Source: CAD feature listing. Evaluate the final solid. Frame: model axes, mm. A direction names the side the tool comes from. Round coordinates to 2 decimals unless told otherwise and drop trailing zeros. Loops run counter-clockwise (first coordinate to the right, second up) from the corner with the lowest first, then second, coordinate; pieces in that order, holes last. Notation, with made-up numbers: (47, -28.75) -> (92, -28.75) arc R36 ccw to (92, 7.25) -> close; hole circle Ø2 at (6, 52). An arc over 180 degrees is marked (long way). Write item = value, one per line.
from build123d import *

# Parameters (mm, degrees)
SKETCH1_R          = 48.5
SKETCH1_R_2        = 27.5
BASE_EXTRUDE_DEPTH = 8


with BuildPart() as part:
    # Sketch1 → Base-Extrude (new body)
    with BuildSketch(Plane.XY):
        with BuildLine():
            Line((456.811048982, 62.151395165), (445.137482247, 71.222327839))
            ThreePointArc((445.137482247, 71.222327839), (408.071209791, 86.463783058), (368.448599855, 80.442214094))
            ThreePointArc((368.448599855, 80.442214094), (344.491847052, 80.189853314), (327.989727135, 97.558495432))
            Line((327.989727135, 97.558495432), (324.860948055, 106.154745303))
            ThreePointArc((324.860948055, 106.154745303), (311.314649231, 123.808625639), (290.092321086, 130.5))
            Line((290.092321086, 130.5), (269.907678914, 130.5))
            ThreePointArc((269.907678914, 130.5), (248.685350769, 123.808625639), (235.139051945, 106.154745303))
            Line((235.139051945, 106.154745303), (216.970143635, 56.236079987))
            ThreePointArc((216.970143635, 56.236079987), (207.211471113, 49.010466943), (196.743512668, 55.163760308))
            Line((196.743512668, 55.163760308), (157.717167982, 134.93418817))
            ThreePointArc((157.717167982, 134.93418817), (154.682682734, 149.146803503), (158.684274169, 163.117981024))
            Line((158.684274169, 163.117981024), (177.676526384, 196.013526811))
            ThreePointArc((177.676526384, 196.013526811), (178.341640473, 198.731623748), (177.442159587, 201.381408993))
            Line((177.442159587, 201.381408993), (176.401319854, 202.867882182))
            ThreePointArc((176.401319854, 202.867882182), (173.173800521, 204.924038765), (169.437677451, 204.095760221))
            Line((169.437677451, 204.095760221), (-40.150350545, 57.3406431))
            ThreePointArc((-40.150350545, 57.3406431), (-66.172482636, -22.829860749), (3.748206743, -69.899577583))
            Line((3.748206743, -69.899577583), (283.212748636, -54.913923642))
            ThreePointArc((283.212748636, -54.913923642), (313.581700751, -44.721920465), (334.378467222, -20.357095704))
            Line((334.378467222, -20.357095704), (358.334984681, 31.017821778))
            ThreePointArc((358.334984681, 31.017821778), (378.340147503, 51.915487493), (406.933003093, 56.316348886))
            Line((406.933003093, 56.316348886), (452.008963478, 48.368240888))
            ThreePointArc((452.008963478, 48.368240888), (455.745086548, 49.196519432), (457.801243132, 52.424038765))
            Line((457.801243132, 52.424038765), (458.667177938, 57.334999088))
            ThreePointArc((458.667177938, 57.334999088), (458.408675401, 60.001230994), (456.811048982, 62.151395165))
        make_face()
        Circle(SKETCH1_R, mode=Mode.SUBTRACT)
        with Locations((280, 5)):
            Circle(SKETCH1_R_2, mode=Mode.SUBTRACT)
        with BuildLine():
            Line((111.606374318, -24.058460629), (149.106374318, -22.04760795))
            ThreePointArc((149.106374318, -22.04760795), (173.367303133, -7.285468557), (174.447868301, 21.093146726))
            Line((174.447868301, 21.093146726), (136.947868301, 97.743703391))
            ThreePointArc((136.947868301, 97.743703391), (103.233762088, 113.786919013), (80, 84.559910536))
            Line((80, 84.559910536), (80, 5.898501192))
            ThreePointArc((80, 5.898501192), (89.362548965, -15.875235621), (111.606374318, -24.058460629))
        make_face(mode=Mode.SUBTRACT)
    extrude(amount=BASE_EXTRUDE_DEPTH)


solid = part.part
1. Section query B-B (x = 14). Return the cut outline in (y, z), then the cut area to 3 significant figures.
Evaluation:
outline = (-69.35, 0) -> (-46.44, 0) -> (-46.44, 8) -> (-69.35, 8) -> close; (46.44, 0) -> (95.26, 0) -> (95.26, 8) -> (46.44, 8) -> close
area = 574 mm²
2. Section query D-D (x = 92.5). Return the cut outline in (y, z), then the cut area to 3 significant figures.
Evaluation:
outline = (-65.14, 0) -> (-18.47, 0) -> (-18.47, 8) -> (-65.14, 8) -> close; (108.93, 0) -> (150.22, 0) -> (150.22, 8) -> (108.93, 8) -> close
area = 704 mm²
3. Section query A-A (y = -13.5). Return the cut outline in (x, z), then the cut area to 3 significant figures.
Evaluation:
outline = (-68.69, 0) -> (-46.58, 0) -> (-46.58, 8) -> (-68.69, 8) -> close; (46.58, 0) -> (87.12, 0) -> (87.12, 8) -> (46.58, 8) -> close; (168.52, 0) -> (259.65, 0) -> (259.65, 8) -> (168.52, 8) -> close; (300.35, 0) -> (337.58, 0) -> (337.58, 8) -> (300.35, 8) -> close
area = 1,530 mm²
4. Line query: probe 1 along X at (y, z) = (28, 4.25); probe 2 along X at (y, z) = (40, 1.75); probe 3 along Y at (x, z) = (282, 4). Output: solid intervals per line, ascending. Write a range as from..to.
Evaluation:
probe_1 = -64.16..-39.6, 39.6..80, 171.07..264.93, 295.07..356.93
probe_2 = -57.45..-27.43, 27.43..80, 165.2..363.89
probe_3 = -54.98..-22.43, 32.43..130.5
5. Mould query, pull axis Y, two halves, no side actions, for faces 4 (the face through (248.95, 123.99, 3.94)), 5 (the face through (89.12, -15.64, 3.94)), 6 (the face through (103.78, 113.91, 3.94)), 7 (the face through (-66.575, -21.629, 3.944)). Classes: released by +Y, released by -Y, zero draft, split by the parting line, or undercut.
Evaluation:
face_4 = released by +Y
face_5 = undercut
face_6 = undercut
face_7 = split by the parting line
6. Set-up query: faces 1 (the face through (226.18, 81.54, 3.94)), 2 (the face through (173.155, -7.641, 3.944)), 3 (the face through (451.06, 66.62, 3.94)). Return all of +Z, -Z, +X, -X, +Y, -Y with unobstructed straight access to the full face (end or side cutting, diameter ignored); none if empty.
Evaluation:
face_1 = +Z, -Z, +Y
face_2 = +Z, -Z
face_3 = +Z, -Z, +X, +Y
7. Contact query for flat-ended pins moving along their axis: pin 1 Ø3 at (y, z) = (1.5, 2) entering from +X; pin 2 Ø1 at (y, z) = (155, 3.5) entering from -X; pin 3 Ø5 at (x, y) = (221.5, -13) entering from -Z; pin 4 Ø1 at (x, z) = (45, 5) entering from -Y. Output: stop coordinate, or through.
Evaluation:
pin_1 = 345.27
pin_2 = 98.61
pin_3 = 0
pin_4 = -67.71
8. Section query C-C (z = 5.5). Give the number of separate pieces and of enclosed holes in the cut face, then the cut area to 3 significant figures.
Evaluation:
separate_pieces = 1
enclosed_holes = 3
area = 53,400 mm²
